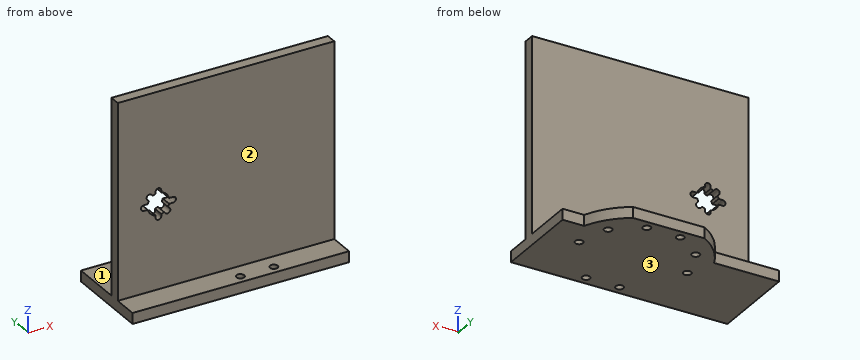
```python
from build123d import *

# Parameters (mm, degrees)
SKETCH2_R           = 1.8
BOSS_EXTRUDE1_DEPTH = 5
SKETCH3_R           = 1.8
BOSS_EXTRUDE2_DEPTH = 5
BOSS_EXTRUDE3_DEPTH = 90
CUT_EXTRUDE3_DEPTH  = 90
CUT_EXTRUDE4_DEPTH  = 90


with BuildPart() as part:
    # Sketch2 → Boss-Extrude1 (new body)
    with BuildSketch(Plane.XY):
        with BuildLine():
            ThreePointArc((30, 52.5), (24.507651866, 61.345374206), (16.5, 68))
            Line((16.5, 68), (-16.5, 68))
            ThreePointArc((-16.5, 68), (-24.507651866, 61.345374206), (-30, 52.5))
            Line((-30, 52.5), (-60, 52.5))
            Line((-60, 52.5), (-60, 12))
            Line((-60, 12), (40, 12))
            Line((40, 12), (40, 52.5))
            Line((40, 52.5), (30, 52.5))
        make_face()
        with Locations((-20.225424859, 25.305368693)):
            Circle(SKETCH2_R, mode=Mode.SUBTRACT)
        with Locations((-25, 40)):
            Circle(SKETCH2_R, mode=Mode.SUBTRACT)
        with Locations((-7.725424859, 16.223587093)):
            Circle(SKETCH2_R, mode=Mode.SUBTRACT)
        with Locations((7.725424859, 16.223587093)):
            Circle(SKETCH2_R, mode=Mode.SUBTRACT)
        with Locations((20.225424859, 25.305368693)):
            Circle(SKETCH2_R, mode=Mode.SUBTRACT)
        with Locations((25, 40)):
            Circle(SKETCH2_R, mode=Mode.SUBTRACT)
        with Locations((-20.225424859, 54.694631307)):
            Circle(SKETCH2_R, mode=Mode.SUBTRACT)
        with Locations((-7.725424859, 63.776412907)):
            Circle(SKETCH2_R, mode=Mode.SUBTRACT)
        with Locations((7.725424859, 63.776412907)):
            Circle(SKETCH2_R, mode=Mode.SUBTRACT)
        with Locations((20.225424859, 54.694631307)):
            Circle(SKETCH2_R, mode=Mode.SUBTRACT)
    extrude(amount=-BOSS_EXTRUDE1_DEPTH)

    # Sketch3 → Boss-Extrude2 (add)
    with BuildSketch(Plane.XY):
        with Locations((-20.225424859, 25.305368693)):
            Circle(SKETCH3_R)
        with Locations((20.225424859, 25.305368693)):
            Circle(SKETCH3_R)
    extrude(amount=-BOSS_EXTRUDE2_DEPTH)

    # Sketch4 → Boss-Extrude3 (add)
    with BuildSketch(Plane.XY):
        Polygon((15.062255845, 23.611), (32.664455845, 23.611), (40, 23.611), (40, 28.611), (-60, 28.611), (-60, 23.611), align=None)
    extrude(amount=BOSS_EXTRUDE3_DEPTH)

    # Sketch5 → Cut-Extrude3 (cut)
    with BuildSketch(Plane(origin=(0, 28.611, 0), x_dir=(1, 0, 0), z_dir=(0, 1, 0))):
        with BuildLine():
            Line((-36.502474055, -39.8011), (-34.402651893, -39.8011))
            ThreePointArc((-34.402651893, -39.8011), (-33.402651893, -38.8011), (-34.402651893, -37.8011))
            Line((-34.402651893, -37.8011), (-36.502474055, -37.8011))
            ThreePointArc((-36.502474055, -37.8011), (-36.762530137, -36.964219525), (-37.170406577, -36.188568247))
            Line((-37.170406577, -36.188568247), (-36.323206271, -35.341367941))
            ThreePointArc((-36.323206271, -35.341367941), (-36.323206271, -33.927154379), (-37.737419834, -33.927154379))
            Line((-37.737419834, -33.927154379), (-38.584620139, -34.774354684))
            ThreePointArc((-38.584620139, -34.774354684), (-39.360271417, -34.366478244), (-40.197151893, -34.106422162))
            Line((-40.197151893, -34.106422162), (-40.197151893, -32.9083))
            ThreePointArc((-40.197151893, -32.9083), (-41.197151893, -31.9083), (-42.197151893, -32.9083))
            Line((-42.197151893, -32.9083), (-42.197151893, -34.106422162))
            ThreePointArc((-42.197151893, -34.106422162), (-44.591264443, -35.40698745), (-45.891829731, -37.8011))
            Line((-45.891829731, -37.8011), (-47.991651893, -37.8011))
            ThreePointArc((-47.991651893, -37.8011), (-48.991651893, -38.8011), (-47.991651893, -39.8011))
            Line((-47.991651893, -39.8011), (-45.891829731, -39.8011))
            ThreePointArc((-45.891829731, -39.8011), (-45.631773649, -40.637980475), (-45.223897209, -41.413631753))
            Line((-45.223897209, -41.413631753), (-46.071097514, -42.260832059))
            ThreePointArc((-46.071097514, -42.260832059), (-46.071097514, -43.675045621), (-44.656883952, -43.675045621))
            Line((-44.656883952, -43.675045621), (-43.809683646, -42.827845316))
            ThreePointArc((-43.809683646, -42.827845316), (-43.034032368, -43.235721756), (-42.197151893, -43.495777838))
            Line((-42.197151893, -43.495777838), (-42.197151893, -44.6939))
            ThreePointArc((-42.197151893, -44.6939), (-41.197151893, -45.6939), (-40.197151893, -44.6939))
            Line((-40.197151893, -44.6939), (-40.197151893, -43.495777838))
            ThreePointArc((-40.197151893, -43.495777838), (-37.803039343, -42.19521255), (-36.502474055, -39.8011))
        make_face()
    extrude(amount=-CUT_EXTRUDE3_DEPTH, mode=Mode.SUBTRACT)

    # Sketch6 → Cut-Extrude4 (cut)
    with BuildSketch(Plane(origin=(0, 28.611, 0), x_dir=(1, 0, 0), z_dir=(0, 1, 0))):
        with BuildLine():
            Line((-37.949551868, -33.715022344), (-38.629271554, -34.39474203))
            ThreePointArc((-38.629271554, -34.39474203), (-39.245466388, -34.089314384), (-39.897151893, -33.869568798))
            Line((-39.897151893, -33.869568798), (-39.897151893, -32.9083))
            ThreePointArc((-39.897151893, -32.9083), (-41.197151893, -31.6083), (-42.497151893, -32.9083))
            Line((-42.497151893, -32.9083), (-42.497151893, -33.869568798))
            ThreePointArc((-42.497151893, -33.869568798), (-44.803396477, -35.194855416), (-46.128683095, -37.5011))
            Line((-46.128683095, -37.5011), (-47.991651893, -37.5011))
            ThreePointArc((-47.991651893, -37.5011), (-49.291651893, -38.8011), (-47.991651893, -40.1011))
            Line((-47.991651893, -40.1011), (-46.128683095, -40.1011))
            ThreePointArc((-46.128683095, -40.1011), (-45.908937509, -40.752785505), (-45.603509863, -41.368980339))
            Line((-45.603509863, -41.368980339), (-46.283229549, -42.048700025))
            ThreePointArc((-46.283229549, -42.048700025), (-46.283229549, -43.887177656), (-44.444751917, -43.887177656))
            Line((-44.444751917, -43.887177656), (-43.765032232, -43.20745797))
            ThreePointArc((-43.765032232, -43.20745797), (-43.148837398, -43.512885616), (-42.497151893, -43.732631202))
            Line((-42.497151893, -43.732631202), (-42.497151893, -44.6939))
            ThreePointArc((-42.497151893, -44.6939), (-41.197151893, -45.9939), (-39.897151893, -44.6939))
            Line((-39.897151893, -44.6939), (-39.897151893, -43.732631202))
            ThreePointArc((-39.897151893, -43.732631202), (-37.590907309, -42.407344584), (-36.26562069, -40.1011))
            Line((-36.26562069, -40.1011), (-34.402651893, -40.1011))
            ThreePointArc((-34.402651893, -40.1011), (-33.102651893, -38.8011), (-34.402651893, -37.5011))
            Line((-34.402651893, -37.5011), (-36.26562069, -37.5011))
            ThreePointArc((-36.26562069, -37.5011), (-36.485366277, -36.849414495), (-36.790793922, -36.233219661))
            Line((-36.790793922, -36.233219661), (-36.111074237, -35.553499975))
            ThreePointArc((-36.111074237, -35.553499975), (-36.111074237, -33.715022344), (-37.949551868, -33.715022344))
        make_face()
    extrude(amount=-CUT_EXTRUDE4_DEPTH, mode=Mode.SUBTRACT)


solid = part.part
```
The model under review builds one solid part; all positions refer to its coordinate system, in mm. Face numbers are marked on the shaded views. A direction names the side the tool comes from. Coordinates: 2 decimals unless noted, no trailing zeros. Write each loop counter-clockwise with the first axis right and the second up, starting at its lowest first coordinate (ties: lowest second). Pieces come first, ordered by that corner, then holes.
1) We need section B-B on x = -25. State the section outline as (y, z) points, then the cut area to 3 significant figures.
2) Machinability: for the marked faces 1, 2 and 3, which of the approach directions +Z, -Z, +X, -X, +Y, -Y give a long, thin tool a straight path to every point of the face, cutting with its end or side? Answer none if there is none.
3) Clearance check with flat-ended pins moving along their axes: pin 1 Ø3 at (x, y) = (20.23, 54.69) entering from +Z; pin 2 Ø5 at (x, z) = (12, 7) entering from +Y; pin 3 Ø6 at (x, y) = (-25, 40) entering from +Z; pin 4 Ø6 at (x, z) = (-3.5, 50) entering from -Y. State where each tip first meets the part, or that it passes through.
4) To check wall thickness, follow probe 1 along Z at (x, y) = (-47.5, 24.5); probe 2 along Y at (x, z) = (13, 79); probe 3 along Z at (x, y) = (-12, 51.5). State the ranges of each line that lie inside material, in increasing order.
5) We need section C-C on x = 14.5. State the section outline as (y, z) points.
6) We need section D-D on z = 30. State the section outline as (x, y) points.
7) We need section A-A on y = 40. State the section outline as (x, z) points.
Answer list:
1. outline: (12, -5) - (38.2, -5) - (38.2, 0) - (28.61, 0) - (28.61, 90) - (23.61, 90) - (23.61, 0) - (12, 0) - close; (41.8, -5) - (60.77, -5) - (60.77, 0) - (41.8, 0) - close
1. area: 676 mm2
2. face 1: +Z, +X, -X, +Y
2. face 2: +Z, +X, -X, -Y
2. face 3: -Z, +X, -X, +Y, -Y
3. pin 1: passes through
3. pin 2: stops at y = 28.61
3. pin 3: stops at z = 0
3. pin 4: stops at y = 23.61
4. probe 1: z = -5 to 37.5, 40.1 to 90
4. probe 2: y = 23.61 to 28.61
4. probe 3: z = -5 to 0
5. outline: (12, -5) - (68, -5) - (68, 0) - (28.61, 0) - (28.61, 90) - (23.61, 90) - (23.61, 0) - (12, 0) - close
6. outline: (-60, 23.61) - (40, 23.61) - (40, 28.61) - (-60, 28.61) - close
7. outline: (-60, -5) - (-26.8, -5) - (-26.8, 0) - (-60, 0) - close; (-23.2, -5) - (23.2, -5) - (23.2, 0) - (-23.2, 0) - close; (26.8, -5) - (40, -5) - (40, 0) - (26.8, 0) - close
